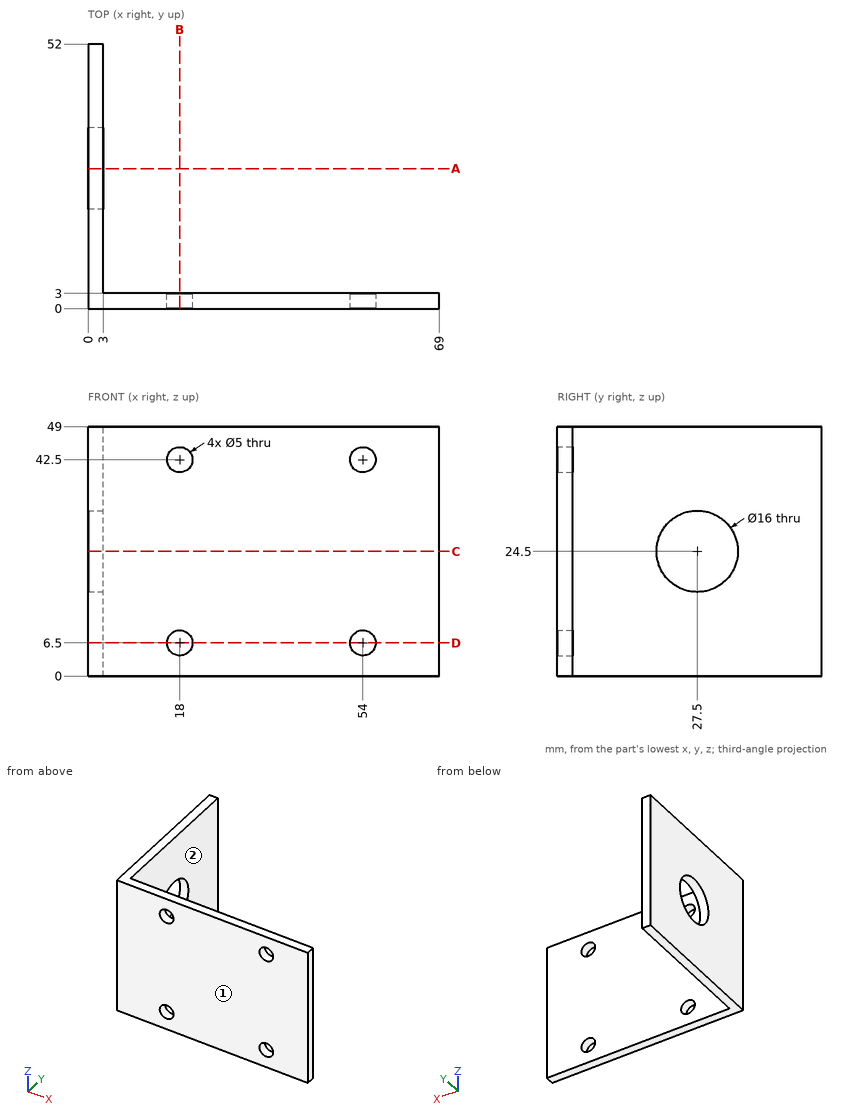
Check sheet for the drawn part. Datum: minimum x, y, z corner. Units: mm. A direction names the side the tool comes from. Give positions to 0.01 mm unless a question says otherwise; leave off trailing zeros. Order: outer loops, then holes, each group sorted by start corner. A loop starts at its lowest first (then second) coordinate and runs counter-clockwise, first axis right, second up. Notation, with made-up numbers: (73, -16.5) -> (123, -16.5) arc R20 cw to (123, -10.5) -> close; hole circle Ø8 at (85, -18). An arc over 180 degrees is marked (long way). Use a Markdown table: item, result.
1) Section check A-A, the plane y = 27.5. Record the boundary of the cut face in (x, z), then the cut area to 3 significant figures.
Results:
| item | result |
|---|---|
| outline | (0, 0) -> (3, 0) -> (3, 16.5) -> (0, 16.5) -> close; (0, 32.5) -> (3, 32.5) -> (3, 49) -> (0, 49) -> close |
| area | 99.0 mm² |
2) Tool access check on the marked faces 1 and 2. Record the directions out of +Z, -Z, +X, -X, +Y, -Y that give a thin tool (end or side, any length) a straight path to the whole face; none if there is none.
Results:
| item | result |
|---|---|
| face 1 | +Z, -Z, +X, -X, -Y |
| face 2 | +Z, -Z, +X, +Y |
3) Section check B-B, the plane x = 18. Record the boundary of the cut face in (y, z), then the cut area to 3 significant figures.
Results:
| item | result |
|---|---|
| outline | (0, 0) -> (3, 0) -> (3, 4) -> (0, 4) -> close; (0, 9) -> (3, 9) -> (3, 40) -> (0, 40) -> close; (0, 45) -> (3, 45) -> (3, 49) -> (0, 49) -> close |
| area | 117 mm² |
4) Section check D-D, the plane z = 6.5. Record the boundary of the cut face in (x, y).
Results:
| item | result |
|---|---|
| outline | (0, 0) -> (15.5, 0) -> (15.5, 3) -> (3, 3) -> (3, 52) -> (0, 52) -> close; (20.5, 0) -> (51.5, 0) -> (51.5, 3) -> (20.5, 3) -> close; (56.5, 0) -> (69, 0) -> (69, 3) -> (56.5, 3) -> close |
5) Material ranges on probe 1 along Z at (x, y) = (18, 1); probe 2 along X at (y, z) = (1.5, 6.5); probe 3 along X at (y, z) = (1, 6), recorded low to high.
Results:
| item | result |
|---|---|
| probe 1 | 0 to 4, 9 to 40, 45 to 49 |
| probe 2 | 0 to 15.5, 20.5 to 51.5, 56.5 to 69 |
| probe 3 | 0 to 15.55, 20.45 to 51.55, 56.45 to 69 |
6) Section check C-C, the plane z = 24.5. Record the boundary of the cut face in (x, y).
Results:
| item | result |
|---|---|
| outline | (0, 0) -> (69, 0) -> (69, 3) -> (3, 3) -> (3, 19.5) -> (0, 19.5) -> close; (0, 35.5) -> (3, 35.5) -> (3, 52) -> (0, 52) -> close |
7) Depth check by flat-ended pin: pin 1 Ø6 at (x, z) = (18, 42.5) entering from +Y; pin 2 Ø10 at (x, y) = (21.5, 7.5) entering from -Z; pin 3 Ø18.5 at (y, z) = (27.5, 24.5) entering from +X; pin 4 Ø3 at (x, z) = (54, 6.5) entering from -Y. Enter the tip coordinate at first touch or a pass-through.
Results:
| item | result |
|---|---|
| pin 1 | y = 3 |
| pin 2 | z = 0 |
| pin 3 | x = 3 |
| pin 4 | through |
